from build123d import *

# Parameters (mm, degrees)
F0_R     = 1.5
F1_DEPTH = 4
F2_R     = 2
F3_R     = 1
F4_R     = 3
F5_W     = 12.076094228
F5_H     = 2
F6_DEPTH = 2
F8_DEPTH = 0.2
F9_R     = 1


with BuildPart() as f1:
    # F0 (on Top) → F1 (new body)
    with BuildSketch(Plane.XY):
        Polygon((0, 19.8), (-2.75, 16.6034741081), (-2.75, -1.4034741081), (0, -4.6), (21.5, -4.6), (24.25, -1.4034741081), (24.25, 16.6034741081), (21.5, 19.8), align=None)
        Circle(F0_R, mode=Mode.SUBTRACT)
        with Locations((21.5, 0)):
            Circle(F0_R, mode=Mode.SUBTRACT)
        with Locations((0, 15.2)):
            Circle(F0_R, mode=Mode.SUBTRACT)
        with BuildLine():
            Line((20.6041763566, -2.6), (0.8958236434, -2.6))
            ThreePointArc((0.8958236434, -2.6), (2.712240771, 0.4541475531), (0, 2.75))
            Line((0, 2.75), (0, 12.45))
            ThreePointArc((0, 12.45), (2.712240771, 14.7458524469), (0.8958236434, 17.8))
            Line((0.8958236434, 17.8), (20.6041763566, 17.8))
            ThreePointArc((20.6041763566, 17.8), (18.787759229, 14.7458524469), (21.5, 12.45))
            Line((21.5, 12.45), (21.5, 2.75))
            ThreePointArc((21.5, 2.75), (18.787759229, 0.4541475531), (20.6041763566, -2.6))
        make_face(mode=Mode.SUBTRACT)
        with Locations((21.5, 15.2)):
            Circle(F0_R, mode=Mode.SUBTRACT)
    extrude(amount=F1_DEPTH)

    # F2
    f2_edges = [f1.edges().sort_by_distance(p)[0] for p in [
        (0.895824, 17.8, 2),
        (20.604176, 17.8, 2),
        (0.895824, -2.6, 2),
        (20.604176, -2.6, 2),
    ]]
    fillet(f2_edges, radius=F2_R)

    # F3
    f3_edges = [f1.edges().sort_by_distance(p)[0] for p in [
        (0, 12.45, 2),
        (0, 2.75, 2),
        (21.5, 12.45, 2),
        (21.5, 2.75, 2),
    ]]
    fillet(f3_edges, radius=F3_R)

    # F4
    f4_edges = [f1.edges().sort_by_distance(p)[0] for p in [
        (0, -4.6, 2),
        (21.5, -4.6, 2),
        (24.25, -1.403474, 2),
        (24.25, 16.603474, 2),
        (21.5, 19.8, 2),
        (0, 19.8, 2),
        (-2.75, 16.603474, 2),
        (-2.75, -1.403474, 2),
    ]]
    fillet(f4_edges, radius=F4_R)

    # F5 (on face) → F6 (cut)
    with BuildSketch(Plane(origin=(0, 0, 0), x_dir=(1, 0, 0), z_dir=(0, 0, -1))):
        with Locations((10.75, -18.8)):
            Rectangle(F5_W, F5_H)
        with BuildLine():
            Line((3.211952886, 4.6), (3.211952886, 1.9228756555))
            ThreePointArc((3.211952886, 1.9228756555), (3.8890772305, 2.4228756555), (4.711952886, 2.6))
            Line((4.711952886, 2.6), (16.788047114, 2.6))
            ThreePointArc((16.788047114, 2.6), (17.6109227695, 2.4228756555), (18.288047114, 1.9228756555))
            Line((18.288047114, 1.9228756555), (18.288047114, 4.6))
            Line((18.288047114, 4.6), (3.211952886, 4.6))
        make_face()
    extrude(amount=-F6_DEPTH, mode=Mode.SUBTRACT)

    # F7 (on face) → F8 (join)
    with BuildSketch(Plane.XY.offset(4)):
        with BuildLine():
            ThreePointArc((-3.5403469074, 18.7514628281), (-4.4378424961, 17.2295966359), (-4.75, 15.4905932629))
            Line((-4.75, 15.4905932629), (-4.75, -0.2905932629))
            ThreePointArc((-4.75, -0.2905932629), (-4.4378424961, -2.0295966359), (-3.5403469074, -3.5514628281))
            Line((-3.5403469074, -3.5514628281), (-2.4138525042, -4.8608695652))
            ThreePointArc((-2.4138525042, -4.8608695652), (-0.7086497373, -6.1444662957), (1.3764944032, -6.6))
            Line((1.3764944032, -6.6), (20.1235055968, -6.6))
            ThreePointArc((20.1235055968, -6.6), (22.2086497373, -6.1444662957), (23.9138525042, -4.8608695652))
            Line((23.9138525042, -4.8608695652), (25.0403469074, -3.5514628281))
            ThreePointArc((25.0403469074, -3.5514628281), (25.9378424961, -2.0295966359), (26.25, -0.2905932629))
            Line((26.25, -0.2905932629), (26.25, 15.4905932629))
            ThreePointArc((26.25, 15.4905932629), (25.9378424961, 17.2295966359), (25.0403469074, 18.7514628281))
            Line((25.0403469074, 18.7514628281), (23.9138525042, 20.0608695652))
            ThreePointArc((23.9138525042, 20.0608695652), (22.2086497373, 21.3444662957), (20.1235055968, 21.8))
            Line((20.1235055968, 21.8), (1.3764944032, 21.8))
            ThreePointArc((1.3764944032, 21.8), (-0.7086497373, 21.3444662957), (-2.4138525042, 20.0608695652))
            Line((-2.4138525042, 20.0608695652), (-3.5403469074, 18.7514628281))
        make_face()
        with BuildLine():
            Line((-2.75, -0.2905932629), (-2.75, 15.4905932629))
            ThreePointArc((-2.75, 15.4905932629), (-2.5627054977, 16.5339952867), (-2.0242081445, 17.447115002))
            Line((-2.0242081445, 17.447115002), (-0.8977137412, 18.7565217391))
            ThreePointArc((-0.8977137412, 18.7565217391), (0.1254079189, 19.5266797774), (1.3764944032, 19.8))
            Line((1.3764944032, 19.8), (20.1235055968, 19.8))
            ThreePointArc((20.1235055968, 19.8), (21.3745920811, 19.5266797774), (22.3977137412, 18.7565217391))
            Line((22.3977137412, 18.7565217391), (23.5242081445, 17.447115002))
            ThreePointArc((23.5242081445, 17.447115002), (24.0627054977, 16.5339952867), (24.25, 15.4905932629))
            Line((24.25, 15.4905932629), (24.25, -0.2905932629))
            ThreePointArc((24.25, -0.2905932629), (24.0627054977, -1.3339952867), (23.5242081445, -2.247115002))
            Line((23.5242081445, -2.247115002), (22.3977137412, -3.5565217391))
            ThreePointArc((22.3977137412, -3.5565217391), (21.3745920811, -4.3266797774), (20.1235055968, -4.6))
            Line((20.1235055968, -4.6), (1.3764944032, -4.6))
            ThreePointArc((1.3764944032, -4.6), (0.1254079189, -4.3266797774), (-0.8977137412, -3.5565217391))
            Line((-0.8977137412, -3.5565217391), (-2.0242081445, -2.247115002))
            ThreePointArc((-2.0242081445, -2.247115002), (-2.5627054977, -1.3339952867), (-2.75, -0.2905932629))
        make_face(mode=Mode.SUBTRACT)
    extrude(amount=-F8_DEPTH)

    # F9
    f9_edges = [f1.edges().sort_by_distance(p)[0] for p in [
        (3.211953, -3.261438, 2),
        (18.288047, -3.261438, 2),
        (16.788047, 18.8, 2),
        (4.711953, 18.8, 2),
    ]]
    fillet(f9_edges, radius=F9_R)


solid = f1.part
The listing builds one solid part. Answer for the finished solid, in the listing's coordinates (mm). A direction names the side the tool comes from. Coordinates: 2 decimals unless noted, no trailing zeros. Write each loop counter-clockwise with the first axis right and the second up, starting at its lowest first coordinate (ties: lowest second). Pieces come first, ordered by that corner, then holes. Notation, with made-up numbers: (62, -20.5) - (95, -20.5) arc R24 ccw to (95, -1.5) - close; hole circle Ø3 at (-39, -30.75). An arc over 180 degrees is marked (long way). Put each result on its own line as item: value.
1. The part is cut by section B-B on x = 6.5. Give the vertices of the cut face in (y, z).
Answer sheet:
outline: (-6.6, 3.8) - (-4.6, 3.8) - (-4.6, 2) - (-2.6, 2) - (-2.6, 4) - (-6.6, 4) - close; (17.8, 2) - (19.8, 2) - (19.8, 3.8) - (21.8, 3.8) - (21.8, 4) - (17.8, 4) - close
2. A tool of negligible diameter and unlimited length cuts with its end or side. For faces 5 (the face through (-2.568, -1.32, 1.927)), 6 (the face through (11, -4, 2)), 7 (the face through (16.788, 18.8, 0.5)), 8 (the face through (22, 8, 0)), 9 (the face through (18.305, 17.104, 2.028)), from which of +Z, -Z, +X, -X, +Y, -Y can it reach the whole face along a straight path? Write none if from no direction.
Answer sheet:
face 5: -Z, -X, -Y
face 6: -Z, -Y
face 7: -Z, +Y, -Y
face 8: -Z, +X, -X, +Y, -Y
face 9: +Z, -Z
3. The part is cut by section A-A on y = 10.75. Give the vertices of the cut face in (x, z), plus the area to 3 significant figures.
Answer sheet:
outline: (-4.75, 3.8) - (-2.75, 3.8) - (-2.75, 0) - (0, 0) - (0, 4) - (-4.75, 4) - close; (21.5, 0) - (24.25, 0) - (24.25, 3.8) - (26.25, 3.8) - (26.25, 4) - (21.5, 4) - close
area: 22.8 mm^2
4. The part is cut by section C-C on z = 0.65. State how many separate pieces and enclosed holes the cut face has, plus the area to 3 significant figures.
Answer sheet:
separate pieces: 2
enclosed holes: 4
area: 174 mm^2
5. Determine the mould class of faces 1 (the face through (-1, 8, 0)), 2 (the face through (2.27, 13.65, 1.97)), 3 (the face through (-2.557, 16.548, 1.927)), 4 (the face through (0.21, 3, 2.03)) for opening direction Y: pulls with the +Y half, pulls with the -Y half, needs draft (parallel to the pull), parting line crosses it, or undercut.
Answer sheet:
face 1: needs draft
face 2: undercut
face 3: pulls with the +Y half
face 4: undercut
6. Flat-ended cylindrical pins translate along their axes: pin 1 Ø0.8 at (y, z) = (-3, 0.5) entering from -X; pin 2 Ø1 at (x, y) = (17, 13) entering from -Z; pin 3 Ø1.1 at (y, z) = (6.5, 1) entering from +X; pin 4 Ø0.8 at (y, z) = (18.5, 0.5) entering from +X. Find the tip coordinate at first contact, or state that the pin passes through.
Answer sheet:
pin 1: stops at x = -1.72
pin 2: passes through
pin 3: stops at x = 24.25
pin 4: stops at x = 22.96
7. Find the intervals of material crossed by line 1 along X through (y, z) = (7, 3.2); line 2 along Y through (x, z) = (8, 3.5); line 3 along X through (y, z) = (16.5, 1.7), in increasing order. Write a range as from..to.
Answer sheet:
line 1: x = -2.75..0, 21.5..24.25
line 2: y = -4.6..-2.6, 17.8..19.8
line 3: x = -2.58..-0.75, 0.75..2.84, 18.66..20.75, 22.25..24.08
